Work out the finished part from the listing and answer in its coordinate system (mm). A direction names the side the tool comes from. Give positions to 0.01 mm unless a question says otherwise; leave off trailing zeros. Write each loop counter-clockwise with the first axis right and the second up, starting at its lowest first coordinate (ties: lowest second). Pieces come first, ordered by that corner, then holes.
1) Find section D-D (y = 17.5). Determine the outline of the cut face in (x, z), plus the area to 3 significant figures.
2) Find section A-A (y = 29). Determine the outline of the cut face in (x, z).
3) Find section B-B (x = 0). Determine the outline of the cut face in (y, z), plus the area to 3 significant figures.
4) Given pin 1 Ø8 at (y, z) = (14, -5) entering from -X; pin 2 Ø6 at (x, z) = (-8.5, -0.5) entering from -Y; pin 3 Ø2.5 at (x, z) = (-1, 0) entering from +Y; pin 4 Ø10 at (y, z) = (24.5, -6.5) entering from +X, each flat-ended and moving along its own axis, determine where each tip first touches the part or whether it passes through.
5) Find section C-C (z = -9). Determine the outline of the cut face in (x, y).
6) A tool of negligible diameter and unlimited length cuts with its end or side. For faces 1 (the face through (0, 43, 11)), 2 (the face through (0, 27, 0)), 3 (the face through (8, 40, -3)), from which of +Z, -Z, +X, -X, +Y, -Y can it reach the whole face along a straight path? Write none if from no direction.
7) Straight lines are drawn through the part: probe 1 along Z at (x, y) = (0, 43.25); probe 2 along Z at (x, y) = (-1.75, 3); probe 3 along Z at (x, y) = (0, 32.75). For each, find the intervals that lie inside material, in ascending order.
```python
from build123d import *

# Parameters (mm, degrees)
SKETCH2_R             = 19.260759025
CUT_EXTRUDE1_DEPTH    = 50
M6X1_0_TAPPED_HOLE1_D = 5
CHAMFER1_SIZE         = 0.2
CHAMFER1_SIZE_2       = 0.169882553
BOSS_EXTRUDE1_START   = -27
SKETCH6_R             = 2.5
BOSS_EXTRUDE1_DEPTH   = 27


with BuildPart() as part:
    # Sketch3 → Revolve1 (revolve)
    with BuildSketch(Plane.XY, mode=Mode.PRIVATE) as revolve1_sk:
        with BuildLine():
            Line((0, 0), (8, 0))
            Line((8, 0), (8, 38))
            ThreePointArc((8, 38), (7, 39), (8, 40))
            Line((8, 40), (12.7, 40))
            ThreePointArc((12.7, 40), (8.980256121, 48.980256121), (0, 52.7))
            Line((0, 52.7), (0, 0))
        make_face()
    revolve(revolve1_sk.sketch.rotate(Axis((0, 0, 0), (0, 1, 0)), 90), axis=Axis((0, 0, 0), (0, 1, 0)))

    # Sketch2 → Cut-Extrude1 (cut)
    with BuildSketch(Plane(origin=(0, 0, 0), x_dir=(1, 0, 0), z_dir=(0, 1, 0))):
        Circle(SKETCH2_R)
        Polygon((-6.350852961, 11), (-12.701705922, 0), (-6.350852961, -11), (6.350852961, -11), (12.701705922, 0), (6.350852961, 11), align=None, mode=Mode.SUBTRACT)
    extrude(amount=CUT_EXTRUDE1_DEPTH, mode=Mode.SUBTRACT)

    # M6x1.0 Tapped Hole1 (through all)
    with Locations(Plane(origin=(0, 0, 0), x_dir=(-1, 0, 0), z_dir=(0, -1, 0))):
        with Locations((0, 0)):
            Hole(M6X1_0_TAPPED_HOLE1_D / 2)

    # Chamfer1
    # the kernel refuses this chamfer: 0.2, 0.169882553 mm, written as the material it takes off along each edge
    with BuildSketch(Plane(origin=(12.957167955, 40, 0.44247322), x_dir=(-0.8660254037844386, 0, 0.5), z_dir=(-0.5000000000000001, 0, -0.8660254037844387)), Plane(origin=(6.095390928, 40, 11.44247322), x_dir=(-0.8660254037844386, 0, -0.5), z_dir=(0.5000000000000001, 0, -0.8660254037844386)), Plane(origin=(-6.861777027, 40, 11), x_dir=(0, 0, -1), z_dir=(1, 0, 0)), Plane(origin=(-12.957167955, 40, -0.44247322), x_dir=(0.8660254037844387, 0, -0.5), z_dir=(0.5, 0, 0.8660254037844387)), Plane(origin=(-6.095390928, 40, -11.44247322), x_dir=(0.8660254037844384, 0, 0.5000000000000002), z_dir=(-0.5000000000000003, 0, 0.8660254037844386)), Plane(origin=(6.861777027, 40, -11), x_dir=(0, 0, 1), z_dir=(-1, 0, 0))) as chamfer1_piece_1:
        Polygon((CHAMFER1_SIZE, 0), (0, CHAMFER1_SIZE), (0, 0), align=None)
    extrude(amount=13.723554053, mode=Mode.SUBTRACT)
    with BuildSketch(Plane(origin=(0, 38, 0), x_dir=(0, 0, -1), z_dir=(1, 0, 0))) as chamfer1_piece_2:
        with BuildLine():
            Line((8, -CHAMFER1_SIZE), (7.774165739, 0.025834261))
            ThreePointArc((7.774165739, 0.025834261), (7.883207603, 0.00684365), (8, 0))
            Line((8, 0), (8, -CHAMFER1_SIZE))
        make_face()
    revolve(axis=Axis((0, 38, 0), (0, 1, 0)), mode=Mode.SUBTRACT)
    with BuildSketch(Plane(origin=(0, 0, 0), x_dir=(0, 0, -1), z_dir=(1, 0, 0))) as chamfer1_piece_3:
        Polygon((8 - CHAMFER1_SIZE, 0), (8, CHAMFER1_SIZE), (8, 0), align=None)
    revolve(axis=Axis((0, 0, 0), (0, 1, 0)), mode=Mode.SUBTRACT)
    with BuildSketch(Plane(origin=(0, 52.451505933, 0), x_dir=(1, 0, 0), z_dir=(0, 0, 1))) as chamfer1_piece_4:
        with BuildLine():
            Line((2.5, -CHAMFER1_SIZE_2), (2.694261242, -0.040585082))
            ThreePointArc((2.694261242, -0.040585082), (2.599956234, -0.020487166), (2.5, 0))
            Line((2.5, 0), (2.5, -CHAMFER1_SIZE_2))
        make_face()
    revolve(axis=Axis((0, 52.451505933, 0), (0, 1, 0)), revolution_arc=90, mode=Mode.SUBTRACT)
    with BuildSketch(Plane(origin=(0, 52.451505933, 0), x_dir=(0, 0, -1), z_dir=(1, 0, 0))) as chamfer1_piece_5:
        with BuildLine():
            Line((2.5, -CHAMFER1_SIZE_2), (2.694261242, -0.040585082))
            ThreePointArc((2.694261242, -0.040585082), (2.599956234, -0.020487166), (2.5, 0))
            Line((2.5, 0), (2.5, -CHAMFER1_SIZE_2))
        make_face()
    revolve(axis=Axis((0, 52.451505933, 0), (0, 1, 0)), revolution_arc=270, mode=Mode.SUBTRACT)

    # Sketch6 → Boss-Extrude1 (add)
    with BuildSketch(Plane.XZ.offset(BOSS_EXTRUDE1_START)):
        with Locations(Location((0, 0, 0), (0, 0, 270))):
            Circle(SKETCH6_R)
    extrude(amount=BOSS_EXTRUDE1_DEPTH)


solid = part.part
```
Results:
1. outline: circle Ø16 at (0, 0)
1. area: 201 mm2
2. outline: circle Ø16 at (0, 0); hole circle Ø5 at (0, 0)
3. outline: (0, -7.8) - (0.2, -8) - (37.8, -8) - (38.03, -7.77) arc R1 cw to (40, -8) - (40, -10.8) - (40.2, -11) - (46.35, -11) arc R12.7 ccw to (52.41, -2.69) - (52.28, -2.5) - (27, -2.5) - (27, 2.5) - (52.28, 2.5) - (52.41, 2.69) arc R12.7 ccw to (46.35, 11) - (40.2, 11) - (40, 10.8) - (40, 8) arc R1 cw to (38.03, 7.77) - (37.8, 8) - (0.2, 8) - (0, 7.8) - close
3. area: 747 mm2
4. pin 1: stops at x = -7.94
4. pin 2: stops at y = 0
4. pin 3: stops at y = 27
4. pin 4: stops at x = 7.86
5. outline: (-7.51, 40.2) - (-7.27, 40) - (7.27, 40) - (7.51, 40.2) - (7.51, 44.89) arc R8.96 ccw to (-7.51, 44.89) - close
6. face 1: +Z, +X, -X, +Y, -Y
6. face 2: +Y
6. face 3: -Y
7. probe 1: z = -11 to -2.5, 2.5 to 11
7. probe 2: z = -7.81 to 7.81
7. probe 3: z = -8 to -2.5, 2.5 to 8
